Check sheet for the modelled part. Datum: model origin and axes. Units: mm. A direction names the side the tool comes from. Round coordinates to 2 decimals unless told otherwise and drop trailing zeros. Order: outer loops, then holes, each group sorted by start corner. A loop starts at its lowest first (then second) coordinate and runs counter-clockwise, first axis right, second up.
Q1. Cross-section at D-D on x = 0. Give the number of separate pieces and of enclosed holes in the cut face, then the cut area to 3 significant figures.
Q2. Mould release check, pull along Y, two halves, no side actions. Record for faces 1 (the flat face through (-21, 1, 4)), 2 (the flat face through (17, 8, -37)), 3 (the cylindrical face through (39.96, 15.6, -1.76)): +Y half, -Y half, draft (parallel to the pull), parting line (faces both ways), or undercut.
Q3. Set-up check for faces 4 (the flat face through (-21.2, 8, -0.5)), 5 (the cylindrical face through (0.44, 3.64, 44.13)), 6 (the cylindrical face through (24.9, 4, 5.5)): record each of +Z, -Z, +X, -X, +Y, -Y from which the full face is reachable in a straight line by a thin tool's end or side.
Q4. Scan lines: probe 1 along Z at (x, y) = (0, 4.2); probe 2 along Y at (x, z) = (42, -18.5); probe 3 along Z at (x, y) = (-8.5, 11.25). Record each from-to range of solid material in increasing order.
Q5. Cross-section at A-A on x = 47.5. Record the cut outline in (y, z) (3 decimals), then the cut area to 3 significant figures.
Q6. Cross-section at C-C on y = 5.25. Record the cut outline in (x, z), then the cut area to 3 significant figures.
Q7. Cross-section at B-B on z = -18.5. Record the cut outline in (x, y), then the cut area to 3 significant figures.
Q8. Depth check by flat-ended pin: P1, Ø1, axis at x = 16.5, y = 11.5, coming from the +Z side; P2, Ø6, axis at y = 15.5, z = -4, coming from the +X side; P3, Ø8, axis at x = 8.5, y = 16, coming from the -Z side. Enter the tip coordinate at first touch or a pass-through.
from build123d import *

# Parameters (mm, degrees)
HOLE_WIZARD_M8_1_D           = 6.8
HOLE_WIZARD_M8_1_CSINK_D     = 8.05
HOLE_WIZARD_M8_1_CSINK_ANGLE = 90
SKETCH_3_R                   = 21
CUT_EXTRUDE_3_DEPTH          = 21


with BuildPart() as part:
    # 草图1 → 旋转1 (revolve)
    with BuildSketch(Plane.XY, mode=Mode.PRIVATE) as revolve_1_sk:
        Polygon((0, 0), (55, 0), (55, 8), (40, 8), (40, 23), (32.5, 23), (32.5, 8), (0, 8), align=None)
    revolve(revolve_1_sk.sketch.rotate(Axis((0, 8, 0), (0, -1, 0)), 180), axis=Axis((0, 8, 0), (0, -1, 0)))

    # M8 螺纹孔1 (through all)
    with Locations(Plane(origin=(0, 8, 0), x_dir=(1, 0, 0), z_dir=(0, 1, 0))):
        with Locations((-47.5, 0), (47.5, 0), (0, -47.5), (0, 47.5)):
            CounterSinkHole(HOLE_WIZARD_M8_1_D / 2, HOLE_WIZARD_M8_1_CSINK_D / 2, counter_sink_angle=HOLE_WIZARD_M8_1_CSINK_ANGLE)

    # 草图3 → 切除-拉伸3 (cut)
    with BuildSketch(Plane(origin=(0, 0, 0), x_dir=(1, 0, 0), z_dir=(0, 1, 0))):
        Circle(SKETCH_3_R)
    extrude(amount=CUT_EXTRUDE_3_DEPTH, mode=Mode.SUBTRACT)

    # 草图4 → 切除-旋转2 (revolve, cut)
    with BuildSketch(Plane(origin=(0, 0, 0), x_dir=(0, 0, -1), z_dir=(1, 0, 0))):
        Polygon((10.5, 7), (10.5, 1), (21, 1), (25.5, 1), (25.5, 4), (25.5, 7), (21, 7), align=None)
    revolve(axis=Axis((0, 0, 0), (0, 1, 0)), mode=Mode.SUBTRACT)


solid = part.part
Results found:
1. separate pieces: 4
1. enclosed holes: 0
1. area: 605 mm2
2. face 1: undercut
2. face 2: +Y half
2. face 3: draft
3. face 4: +Y
3. face 5: +Y, -Y
3. face 6: none
4. probe 1: z = -55 to -50.9, -44.1 to -25.5, 25.5 to 44.1, 50.9 to 55
4. probe 2: y = 0 to 8
4. probe 3: z = -39.09 to -31.37, 31.37 to 39.09
5. outline: (0, -27.726) - (8, -27.726) - (8, -4.025) - (7.375, -3.4) - (0, -3.4) - close; (0, 3.4) - (7.375, 3.4) - (8, 4.025) - (8, 27.726) - (0, 27.726) - close
5. area: 389 mm2
6. outline: circle Ø110 at (0, 0); hole circle Ø6.8 at (-47.5, 0); hole circle Ø51 at (0, 0); hole circle Ø6.8 at (0, -47.5); hole circle Ø6.8 at (0, 47.5); hole circle Ø6.8 at (47.5, 0)
6. area: 7,320 mm2
7. outline: (-51.8, 0) - (-9.94, 0) - (-9.94, 1) - (-17.55, 1) - (-17.55, 7) - (-9.94, 7) - (-9.94, 8) - (-26.72, 8) - (-26.72, 23) - (-35.46, 23) - (-35.46, 8) - (-51.8, 8) - close; (9.94, 0) - (51.8, 0) - (51.8, 8) - (35.46, 8) - (35.46, 23) - (26.72, 23) - (26.72, 8) - (9.94, 8) - (9.94, 7) - (17.55, 7) - (17.55, 1) - (9.94, 1) - close
7. area: 841 mm2
8. P1: stops at z = 36.66
8. P2: stops at x = 39.99
8. P3: stops at z = -39.75
